Autodesk Inventor part; units mm, degrees
ref_plane "YZ Plane" through (0, 0, 0) normal (1, 0, 0) x (0, 1, 0)
ref_plane "XZ Plane" through (0, 0, 0) normal (0, 1, 0) x (-1, 0, 0)
ref_plane "XY Plane" through (0, 0, 0) normal (0, 0, 1) x (1, 0, 0)
sketch "Sketch1" plane through (0, 0, 0) normal (0, 1, 0) x (-1, 0, 0)
  line L0 (0, 0) -> (220, 0)
  line L1 (220, 0) -> (220, 70)
  line L2 (220, 70) -> (0, 70)
  line L3 (0, 70) -> (0, 0)
  dimension "d11" = 220
  dimension "d16" = 70
extrude "Extrusion3" add sketch "Sketch1" along normal blind 6
sketch "Sketch5" plane through (0, 0, 0) normal (0, -1, 0) x (1, 0, 0)
  line L0 (0, 0) -> (-220, 0)
  line L1 (0, 70) -> (0, 0)
  line L2 (-220, 70) -> (0, 70)
  line L3 (-220, 0) -> (-220, 70)
  line L4 (-220, 55) -> (-224, 55)
  line L5 (-226, 53) -> (-226, 49)
  line L6 (-224, 47) -> (-220, 47)
  line L7 (-220, 47) -> (-220, 55)
  line L8 (-220, 23) -> (-224, 23)
  line L9 (-226, 21) -> (-226, 17)
  line L10 (-224, 15) -> (-220, 15)
  line L11 (-220, 15) -> (-220, 23)
  line L12 (0, 55) -> (4, 55)
  line L13 (6, 53) -> (6, 49)
  line L14 (4, 47) -> (0, 47)
  line L15 (0, 47) -> (0, 55)
  line L16 (0, 23) -> (4, 23)
  line L17 (6, 21) -> (6, 17)
  line L18 (4, 15) -> (0, 15)
  line L19 (0, 15) -> (0, 23)
  arc A0 (-224, 55) -> (-226, 53) centre (-224, 53) ccw
  arc A1 (-226, 49) -> (-224, 47) centre (-224, 49) ccw
  arc A2 (-224, 23) -> (-226, 21) centre (-224, 21) ccw
  arc A3 (-226, 17) -> (-224, 15) centre (-224, 17) ccw
  arc A4 (4, 47) -> (6, 49) centre (4, 49) ccw
  arc A5 (6, 53) -> (4, 55) centre (4, 53) ccw
  arc A6 (6, 21) -> (4, 23) centre (4, 21) ccw
  arc A7 (4, 15) -> (6, 17) centre (4, 17) ccw
  dimension "d61" = 2
  dimension "d62" = 8
  dimension "d63" = 8
  dimension "d64" = 6
  dimension "d65" = 15
  dimension "d66" = 15
  dimension "d67" = 6
extrude "Extrusion6" add sketch "Sketch5" against normal blind 6 contours L1 L16 A6 L17 A7 L18 | L10 A3 L9 A2 L8 L3 | L1 L12 A5 L13 A4 L14 | L6 A1 L5 A0 L4 L3
sketch "Sketch6" plane through (0, 0, 0) normal (0, -1, 0) x (1, 0, 0)
  line L0 (0, 0) -> (-220, 0)
  line L1 (-220, 70) -> (0, 70)
  line L2 (-220, 23) -> (-220, 47)
  line L3 (-110, 70) -> (-110, 0) construction
  line L4 (-203.7, 37.25) -> (-203.7, 32.75)
  line L5 (-220, 32.75) -> (-220, 37.25)
  line L6 (-215, 39.75) -> (-207.7, 39.75)
  line L7 (-207.7, 30.25) -> (-215, 30.25)
  line L8 (-220, 37.25) -> (-215, 37.25)
  line L9 (-207.7, 37.25) -> (-203.7, 37.25)
  line L10 (-203.7, 32.75) -> (-207.7, 32.75)
  line L11 (-215, 32.75) -> (-220, 32.75)
  line L12 (-215, 30.25) -> (-215, 32.75)
  line L13 (-215, 37.25) -> (-215, 39.75)
  line L14 (-207.7, 39.75) -> (-207.7, 37.25)
  line L15 (-207.7, 32.75) -> (-207.7, 30.25)
  line L16 (-16.3, 37.25) -> (-16.3, 32.75)
  line L17 (0, 32.75) -> (0, 37.25)
  line L18 (-5, 39.75) -> (-12.3, 39.75)
  line L19 (-12.3, 30.25) -> (-5, 30.25)
  line L20 (0, 37.25) -> (-5, 37.25)
  line L21 (-12.3, 37.25) -> (-16.3, 37.25)
  line L22 (-16.3, 32.75) -> (-12.3, 32.75)
  line L23 (-5, 32.75) -> (0, 32.75)
  line L24 (-5, 30.25) -> (-5, 32.75)
  line L25 (-5, 37.25) -> (-5, 39.75)
  line L26 (-12.3, 39.75) -> (-12.3, 37.25)
  line L27 (-12.3, 32.75) -> (-12.3, 30.25)
  point P0 (-220, 35)
  point P1 (0, 35)
  dimension "d70" = 2.5
  dimension "d71" = 2.5
  dimension "d72" = 4.5
  dimension "d73" = 5
  dimension "d74" = 7.3
  dimension "d75" = 4
extrude "Extrusion7" cut sketch "Sketch6" against normal blind 6
equation "\"d66\" = d65"
equation "\"d71\" = d70"
properties part number "front_panel_2004_bottom"
Geometry check sheet. Reference: the model listing, model coordinates, mm. A direction names the side the tool comes from. Round coordinates to 2 decimals unless told otherwise and drop trailing zeros. Loops run counter-clockwise (first coordinate to the right, second up) from the corner with the lowest first, then second, coordinate; pieces in that order, holes last. Notation, with made-up numbers: (41, -2) -> (78, -2) arc R15 cw to (78, 10) -> close; hole circle Ø1 at (-23.5, 23). An arc over 180 degrees is marked (long way). Answer as a JSON object with one key per item and string values. Group by question number.
Item 1: Release check for a two-part mould opening along X. For faces 6 (the face through (-203.7, 3, 35)), 7 (the face through (-9, 3, 30.25)), 8 (the face through (2, 3, 15)) record: pulls with the +X half, pulls with the -X half, needs draft (parallel to the pull), parting line crosses it, or undercut.
Item 2: Cross-section at A-A, the plane z = 26.5. Record the cut outline in (x, y), plus the area to 3 significant figures.
Item 3: Set-up check for faces 1 (the face through (-220, 3, 62)), 2 (the face through (0, 3, 63)), 3 (the face through (-9, 3, 39.75)), 4 (the face through (2, 3, 23)), 5 (the face through (-220, 3, 42)): record each of +Z, -Z, +X, -X, +Y, -Y from which the full face is reachable in a straight line by a thin tool's end or side.
Item 4: Thickness scan on line 1 along X through (y, z) = (3.3, 37.5); line 2 along Z through (x, y) = (-213, 5.5); line 3 along Z through (x, y) = (-14.5, 5.5). Record the ranges inside material, lowest first.
Item 5: Depth check by flat-ended pin: pin 1 Ø3 at (y, z) = (4, 39) entering from +X; pin 2 Ø3 at (x, y) = (2.5, 3.5) entering from +Z; pin 3 Ø1.5 at (x, y) = (-2.5, 4) entering from -Z; pin 4 Ø0.8 at (y, z) = (3, 39) entering from -X. Enter the tip coordinate at first touch or a pass-through.
Determined:
{
 "1": {"face 6": "pulls with the -X half", "face 7": "undercut", "face 8": "needs draft"},
 "2": {"outline": "(-220, 0) -> (0, 0) -> (0, 6) -> (-220, 6) -> close", "area": "1,320 mm²"},
 "3": {"face 1": "+Z, -X, +Y, -Y", "face 2": "+Z, +X, +Y, -Y", "face 3": "+Y, -Y", "face 4": "+X, +Y, -Y", "face 5": "-X, +Y, -Y"},
 "4": {"line 1": "x = -220 to -215, -207.7 to -12.3, -5 to 0", "line 2": "z = 0 to 30.25, 39.75 to 70", "line 3": "z = 0 to 32.75, 37.25 to 70"},
 "5": {"pin 1": "stops at x = 0", "pin 2": "stops at z = 55", "pin 3": "stops at z = 0", "pin 4": "stops at x = -220"}
}
